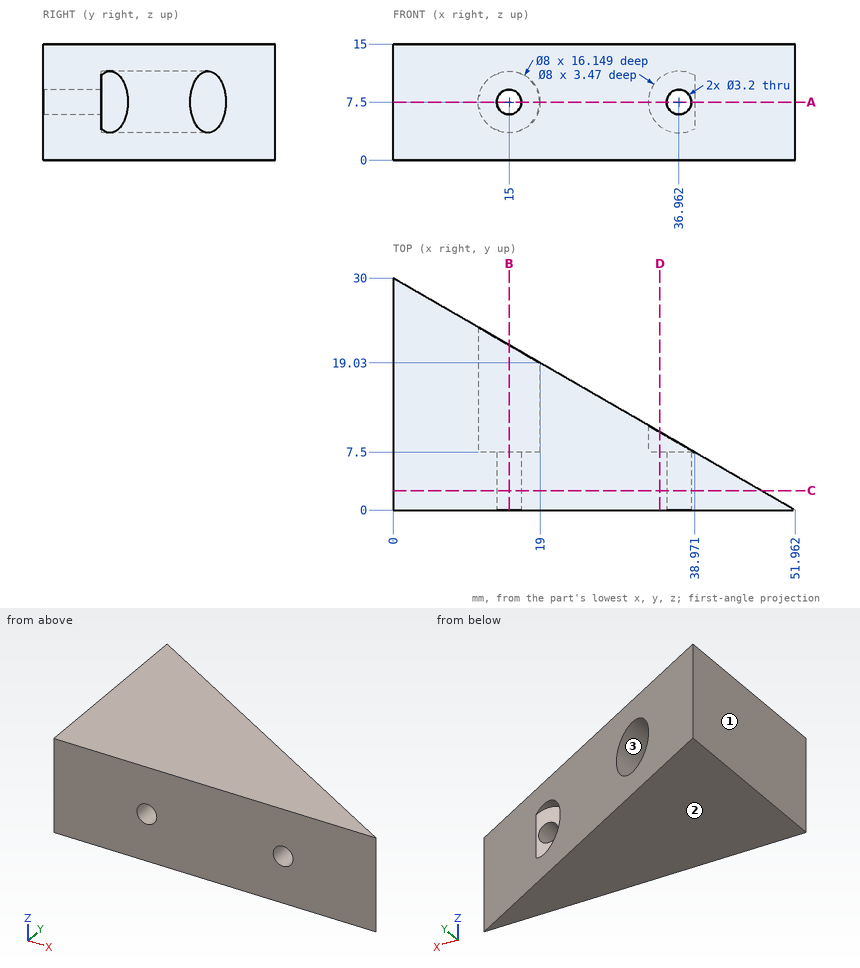
Geometry: see drawing. Coordinates: mm, zero at the bounding-box minimum. Give positions to 0.01 mm unless a question says otherwise; leave off trailing zeros. Loops run counter-clockwise (first coordinate to the right, second up) from the corner with the lowest first, then second, coordinate; pieces in that order, holes last. Notation, with made-up numbers: (30.25, 48.25) -> (78.25, 48.25) arc R10 ccw to (78.25, 55.25) -> close; hole circle Ø10 at (-24, 66.25). An arc over 180 degrees is marked (long way). Put each result on its own line as item: value.
1. Cut plane B-B (x = 15). Return the cut outline in (y, z).
Taken from the geometry:
outline: (0, 0) -> (21.34, 0) -> (21.34, 3.5) -> (7.5, 3.5) -> (7.5, 5.9) -> (0, 5.9) -> close; (0, 9.1) -> (7.5, 9.1) -> (7.5, 11.5) -> (21.34, 11.5) -> (21.34, 15) -> (0, 15) -> close
2. Pin query (flat end, axial travel): P1, Ø5, axis at x = 23.5, z = 12.5, coming from the +Y side (1 decimal); P2, Ø5, axis at x = 36, z = 5.5, coming from the +Y side; P3, Ø4, axis at y = 27, z = 10, coming from the +X side; P4, Ø4, axis at x = 19.5, y = 12, coming from the -Z side. Return the tip coordinate at first contact, or that it passes through.
Taken from the geometry:
P1: stops at y = 17.9
P2: stops at y = 10.66
P3: stops at x = 8.66
P4: stops at z = 0
3. Cut plane D-D (x = 34.5). Return the cut outline in (y, z).
Taken from the geometry:
outline: (0, 0) -> (10.08, 0) -> (10.08, 4.35) -> (7.5, 4.35) -> (7.5, 10.65) -> (10.08, 10.65) -> (10.08, 15) -> (0, 15) -> close
4. Cut plane C-C (y = 2.5). Return the cut outline in (x, z).
Taken from the geometry:
outline: (0, 0) -> (47.63, 0) -> (47.63, 15) -> (0, 15) -> close; hole circle Ø3.2 at (15, 7.5); hole circle Ø3.2 at (36.96, 7.5)
5. Ray query, line 1 along Z through (x, y) = (15, 13); line 2 along X through (y, z) = (1.75, 7.5) (1 decimal); line 3 along X through (y, z) = (3.75, 8) (1 decimal). Return the intervals inside material, ascending. Write a range as [from, to].
Taken from the geometry:
line 1: z = [0, 3.5], [11.5, 15]
line 2: x = [0, 13.4], [16.6, 35.4], [38.6, 48.9]
line 3: x = [0, 13.5], [16.5, 35.4], [38.5, 45.5]
6. Pull-direction query (Z, two-part tool) for the marked faces 1, 2 and 3; classes: released by +Z, released by -Z, zero draft, split by the parting line, or undercut.
Taken from the geometry:
face 1: zero draft
face 2: released by -Z
face 3: undercut
7. Cut plane A-A (z = 7.5). Return the cut outline in (x, y), plus the area to 3 significant figures.
Taken from the geometry:
outline: (0, 0) -> (13.4, 0) -> (13.4, 7.5) -> (11, 7.5) -> (11, 23.65) -> (0, 30) -> close; (16.6, 0) -> (35.36, 0) -> (35.36, 7.5) -> (32.96, 7.5) -> (32.96, 10.97) -> (19, 19.03) -> (19, 7.5) -> (16.6, 7.5) -> close; (38.56, 0) -> (51.96, 0) -> (38.97, 7.5) -> (38.56, 7.5) -> close
area: 610 mm2
